Geometry: final body of the model. Coordinates: model frame, mm. A direction names the side the tool comes from. Give positions to 0.01 mm unless a question says otherwise; leave off trailing zeros. Loops run counter-clockwise (first coordinate to the right, second up) from the corner with the lowest first, then second, coordinate; pieces in that order, holes last.
from build123d import *

# Parameters (mm, degrees)
SKETCH1_W                 = 375
SKETCH1_H                 = 10.632083078
BOSS_EXTRUDE1_DEPTH       = 9.738944775
SKETCH2_W                 = 9.738944775
SKETCH2_H                 = 25
BOSS_EXTRUDE2_DEPTH       = 249.367916922
BOSS_EXTRUDE3_DEPTH       = 0.632083078
SKETCH4_W                 = 489.738944775
SKETCH4_H                 = 375
BOSS_EXTRUDE4_DEPTH       = 30
SKETCH5_W                 = 489.738944775
SKETCH5_H                 = 290.632083078
BOSS_EXTRUDE5_DEPTH       = 25
SKETCH6_W                 = 400
SKETCH6_H                 = 290.632083078
BOSS_EXTRUDE6_DEPTH       = 10.261055225
SKETCH7_W                 = 500
SKETCH7_H                 = 400
BOSS_EXTRUDE7_DEPTH       = 9.367916922
SKETCH8_W                 = 480
SKETCH8_H                 = 260
CUT_EXTRUDE1_DEPTH        = 15
M25_CLEARANCE_HOLE1_D     = 28.660544953
M25_CLEARANCE_HOLE1_DEPTH = 9.367916922
M45_CLEARANCE_HOLE1_D     = 50
M45_CLEARANCE_HOLE1_DEPTH = 9.367916922


with BuildPart() as part:
    # Sketch1 → Boss-Extrude1 (new body)
    with BuildSketch(Plane(origin=(250, 0, 0), x_dir=(0, 0, -1), z_dir=(1, 0, 0))):
        with Locations((-12.5, 285.316041539)):
            Rectangle(SKETCH1_W, SKETCH1_H)
    extrude(amount=-BOSS_EXTRUDE1_DEPTH)

    # Sketch2 → Boss-Extrude2 (add)
    with BuildSketch(Plane.XZ.offset(-280)):
        with Locations((245.130527613, 187.5)):
            Rectangle(SKETCH2_W, SKETCH2_H)
    extrude(amount=BOSS_EXTRUDE2_DEPTH)

    # Sketch3 → Boss-Extrude3 (add)
    with BuildSketch(Plane.XZ.offset(-30.632083078)):
        Polygon((-50, 175), (-50, -175), (-239.738944775, -175), (-239.738944775, 200), (250, 200), (250, 175), align=None)
    extrude(amount=BOSS_EXTRUDE3_DEPTH)

    # Sketch4 → Boss-Extrude4 (add)
    with BuildSketch(Plane.XZ.offset(-30)):
        with Locations((5.130527613, 12.5)):
            Rectangle(SKETCH4_W, SKETCH4_H)
    extrude(amount=BOSS_EXTRUDE4_DEPTH)

    # Sketch5 → Boss-Extrude5 (add)
    with BuildSketch(Plane(origin=(0, 0, -175), x_dir=(-1, 0, 0), z_dir=(0, 0, -1))):
        with Locations((-5.130527613, 145.316041539)):
            Rectangle(SKETCH5_W, SKETCH5_H)
    extrude(amount=BOSS_EXTRUDE5_DEPTH)

    # Sketch6 → Boss-Extrude6 (add)
    with BuildSketch(Plane.ZY.offset(239.738944775)):
        with Locations((0, 145.316041539)):
            Rectangle(SKETCH6_W, SKETCH6_H)
    extrude(amount=BOSS_EXTRUDE6_DEPTH)

    # Sketch7 → Boss-Extrude7 (add)
    with BuildSketch(Plane(origin=(0, 290.632083078, 0), x_dir=(-1, 0, 0), z_dir=(0, 1, 0))):
        Rectangle(SKETCH7_W, SKETCH7_H)
    extrude(amount=BOSS_EXTRUDE7_DEPTH)

    # Sketch8 → Cut-Extrude1 (cut)
    with BuildSketch(Plane.XY.offset(-175)):
        with Locations((0.261055225, 160.632083078)):
            Rectangle(SKETCH8_W, SKETCH8_H)
    extrude(amount=-CUT_EXTRUDE1_DEPTH, mode=Mode.SUBTRACT)

    # M25 Clearance Hole1
    with Locations(Plane(origin=(0, 290.632083078, 0), x_dir=(-1, 0, 0), z_dir=(0, -1, 0))):
        with Locations((-107.763649025, -120.947499703), (120.947499703, -120.947499703)):
            Hole(M25_CLEARANCE_HOLE1_D / 2, depth=M25_CLEARANCE_HOLE1_DEPTH)

    # M45 Clearance Hole1
    with Locations(Plane(origin=(0, 290.632083078, 0), x_dir=(-1, 0, 0), z_dir=(0, -1, 0))):
        with Locations((0, 0)):
            Hole(M45_CLEARANCE_HOLE1_D / 2, depth=M45_CLEARANCE_HOLE1_DEPTH)


solid = part.part
Item 1: Set-up query: faces 1 (the face through (38, 27, 200)), 2 (the face through (245, 156, -175)), 3 (the face through (4, 148, -200)), 4 (the face through (240.261, 286, 47)), 5 (the face through (-114.33, 295.38, 133.66)). Return all of +Z, -Z, +X, -X, +Y, -Y with unobstructed straight access to the full face (end or side cutting, diameter ignored); none if empty.
Values follow:
face 1: +Z, +X, -X, +Y, -Y
face 2: +X
face 3: -Z, +X, -X, +Y, -Y
face 4: +Z
face 5: +Y
Item 2: Draft query along Y for faces 6 (the face through (3, 300, 47)), 7 (the face through (245, 156, 175)), 8 (the face through (4, 0, -3)), 9 (the face through (250, 16, -1)). Return one class per face: +Y half, -Y half, draft (parallel to the pull), parting line (faces both ways), or undercut.
Values follow:
face 6: +Y half
face 7: undercut
face 8: -Y half
face 9: draft
Item 3: Section query C-C on y = 51. Return loops of the section in (x, z), plus the area to 3 significant figures.
Values follow:
outline: (-250, -200) - (250, -200) - (250, -175) - (240.26, -175) - (240.26, -190) - (-239.74, -190) - (-239.74, 200) - (-250, 200) - close; (240.26, 175) - (250, 175) - (250, 200) - (240.26, 200) - close
area: 9,390 mm2
Item 4: Section query B-B on z = 7. Return loops of the section in (x, y).
Values follow:
outline: (-250, 0) - (250, 0) - (250, 30) - (-50, 30) - (-50, 30.63) - (-239.74, 30.63) - (-239.74, 290.63) - (-24, 290.63) - (-24, 300) - (-250, 300) - close; (24, 290.63) - (240.26, 290.63) - (240.26, 280) - (250, 280) - (250, 300) - (24, 300) - close
Item 5: Pin query (flat end, axial travel): pin 1 (4 mm diameter, centred on y = 102.5, z = 128, fed in from +X); pin 2 (8 mm diameter, centred on y = 34.5, z = 33.5, fed in from +X). Return the tip coordinate at first contact, or that it passes through.
Values follow:
pin 1: stops at x = -239.74
pin 2: stops at x = -50
Item 6: Ray query, probe 1 along Y at (x, z) = (-214, 89); probe 2 along Y at (x, z) = (41, 168.5); probe 3 along Z at (x, y) = (0, 295). Return the intervals inside material, ascending.
Values follow:
probe 1: y = 0 to 30.63, 290.63 to 300
probe 2: y = 0 to 30, 290.63 to 300
probe 3: z = -200 to -25, 25 to 200
Item 7: Section query D-D on x = -153. Return loops of the section in (y, z), plus the area to 3 significant figures.
Values follow:
outline: (0, -200) - (300, -200) - (300, 200) - (290.63, 200) - (290.63, -190) - (30.63, -190) - (30.63, 200) - (0, 200) - close
area: 18,600 mm2
Item 8: Section query A-A on x = 0. Return loops of the section in (y, z), plus the area to 3 significant figures.
Values follow:
outline: (0, -200) - (300, -200) - (300, -25) - (290.63, -25) - (290.63, -190) - (30.63, -190) - (30.63, -175) - (30, -175) - (30, 175) - (30.63, 175) - (30.63, 200) - (0, 200) - close; (290.63, 25) - (300, 25) - (300, 200) - (290.63, 200) - close
area: 17,900 mm2
